Can you work these out from the model? Positions are in its coordinate system, mm. Face numbers are marked on the shaded views. Round coordinates to 2 decimals unless told otherwise and drop trailing zeros. Order: outer loops, then holes, each group sorted by start corner. A loop starts at its lowest first (then second) coordinate and runs counter-clockwise, first axis right, second up. Notation, with made-up numbers: (54.5, -10) -> (106.5, -10) arc R8 ccw to (106.5, -2) -> close; hole circle Ø9 at (52, -8.5). An arc over 180 degrees is marked (long way). Use a Markdown table: item, result. Add a question column.
Q1. I'm going to push flat-ended pins straight in: pin 1 Ø2 at (x, y) = (25.575, -43.247) entering from +Z (1 decimal); pin 2 Ø10 at (x, y) = (13, -30) entering from +Z; pin 3 Ø2 at (x, z) = (15, 4.5) entering from +Y. Where does each tip first touch, or does it pass through?
Q2. I need wall thicknesses on line 1 along X through (y, z) = (34.5, 5.5) (3 decimals); line 2 along X through (y, z) = (56.5, 3.25) (3 decimals); line 3 along X through (y, z) = (22.5, 3.5) (3 decimals). Which ranges of each line are inside material? Lowest first, please. Write a range as [from, to].
Q3. If we section it at D-D on z = 2: Give the number of separate pieces and of enclosed holes in the cut face, plus the area to 3 significant figures.
Q4. If we section it at C-C on x = -13: List the corners of the cut face in (y, z) for me.
Q5. If we section it at A-A on x = -3: List the corners of the cut face in (y, z) for me, plus the area to 3 significant figures.
Q6. We'd pull the mould along X, two halves only. Please class the marked faces 1 and 2: +X half, -X half, draft (parallel to the pull), parting line (faces both ways), or undercut.
Q7. If we section it at B-B on y = -59: List the corners of the cut face in (x, z) for me (3 decimals).
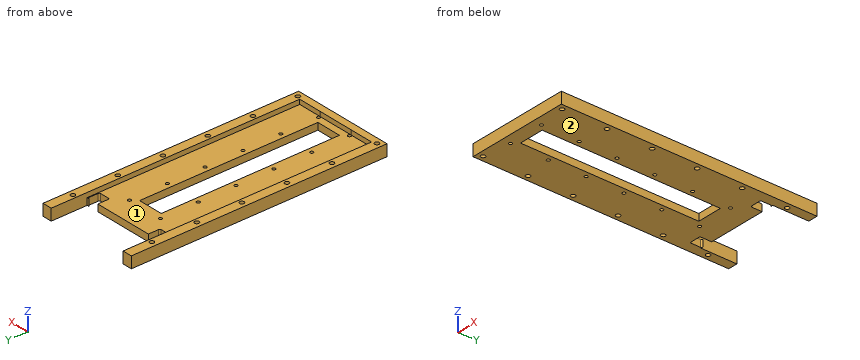
```python
from build123d import *

# Parameters (mm, degrees)
SKETCH1_W                 = 57.15
SKETCH1_H                 = 142.494
BOSS_EXTRUDE1_DEPTH       = 6.35
SKETCH2_W                 = 14
SKETCH2_H                 = 99
CUT_EXTRUDE1_DEPTH        = 78.025892621
SKETCH3_R                 = 1.2192
CUT_EXTRUDE2_DEPTH        = 78.025892621
LPATTERN1_COUNT           = 6
LPATTERN1_PITCH           = 25
LPATTERN1_COPY_1_SKETCH_R = 1.2192
LPATTERN1_COPY_1_DEPTH    = 78.025892621
LPATTERN1_COPY_2_SKETCH_R = 1.2192
LPATTERN1_COPY_2_DEPTH    = 78.025892621
LPATTERN1_COPY_3_SKETCH_R = 1.2192
LPATTERN1_COPY_3_DEPTH    = 78.025892621
LPATTERN1_COPY_4_SKETCH_R = 1.2192
LPATTERN1_COPY_4_DEPTH    = 78.025892621
LPATTERN1_COPY_5_SKETCH_R = 1.2192
LPATTERN1_COPY_5_DEPTH    = 78.025892621
SKETCH4_R                 = 0.889
CUT_EXTRUDE3_DEPTH        = 78.025892621
LPATTERN2_COUNT           = 6
LPATTERN2_PITCH           = 21
LPATTERN2_COPY_1_SKETCH_R = 0.889
LPATTERN2_COPY_1_DEPTH    = 78.025892621
LPATTERN2_COPY_2_SKETCH_R = 0.889
LPATTERN2_COPY_2_DEPTH    = 78.025892621
LPATTERN2_COPY_3_SKETCH_R = 0.889
LPATTERN2_COPY_3_DEPTH    = 78.025892621
LPATTERN2_COPY_4_SKETCH_R = 0.889
LPATTERN2_COPY_4_DEPTH    = 78.025892621
LPATTERN2_COPY_5_SKETCH_R = 0.889
LPATTERN2_COPY_5_DEPTH    = 78.025892621
SKETCH6_W                 = 41.91
SKETCH6_H                 = 10.16
CUT_EXTRUDE4_DEPTH        = 78.025892621
SKETCH8_W                 = 46.5
SKETCH8_H                 = 152.4
CUT_EXTRUDE6_DEPTH        = 2.54
SKETCH9_W                 = 57.15
SKETCH9_H                 = 6.35
CUT_EXTRUDE7_DEPTH        = 0.5
SKETCH11_W                = 6.5
SKETCH11_H                = 6.5
CUT_EXTRUDE8_DEPTH        = 78.025892621
FILLET1_R                 = 0.75
FILLET1_OF_MIRROR4_R      = 0.75
SKETCH12_W                = 41.91
SKETCH12_H                = 9.793222615
CUT_EXTRUDE9_DEPTH        = 77.858192368
SKETCH13_W                = 46.5
SKETCH13_H                = 19.953222615
CUT_EXTRUDE10_DEPTH       = 77.858192368


with BuildPart() as part:
    # Sketch1 → Boss-Extrude1 (new body)
    with BuildSketch(Plane.XY):
        Rectangle(SKETCH1_W, SKETCH1_H)
    extrude(amount=BOSS_EXTRUDE1_DEPTH)

    # Sketch2 → Cut-Extrude1 (cut, through all)
    with BuildSketch(Plane.XY.offset(6.35)):
        with Locations((0, -13.879757445)):
            Rectangle(SKETCH2_W, SKETCH2_H)
    extrude(amount=-CUT_EXTRUDE1_DEPTH, mode=Mode.SUBTRACT)

    # Sketch3 → Cut-Extrude2 (cut, through all)
    with BuildSketch(Plane.XY.offset(6.35)):
        with Locations((-25.575, -68.247)):
            Circle(SKETCH3_R)
    cut_extrude2 = extrude(amount=-CUT_EXTRUDE2_DEPTH, mode=Mode.SUBTRACT)

    # Mirror1: Cut-Extrude2 across plane
    add(cut_extrude2.mirror(Plane(origin=(0, 0, 0), x_dir=(0, 0, 1), z_dir=(1, 0, 0))), mode=Mode.SUBTRACT)

    # LPattern1: Cut-Extrude2 ×6
    with Locations(*[(0, i * LPATTERN1_PITCH, 0) for i in range(1, LPATTERN1_COUNT)]):
        add(cut_extrude2, mode=Mode.SUBTRACT)

    # LPattern1 copy 1 sketch → LPattern1 copy 1 (cut, through all)
    with BuildSketch(Plane(origin=(0, 25, 6.35), x_dir=(-1, 0, 0), z_dir=(0, 0, 1))):
        with Locations((-25.575, 68.247)):
            Circle(LPATTERN1_COPY_1_SKETCH_R)
    extrude(amount=-LPATTERN1_COPY_1_DEPTH, mode=Mode.SUBTRACT)

    # LPattern1 copy 2 sketch → LPattern1 copy 2 (cut, through all)
    with BuildSketch(Plane(origin=(0, 50, 6.35), x_dir=(-1, 0, 0), z_dir=(0, 0, 1))):
        with Locations((-25.575, 68.247)):
            Circle(LPATTERN1_COPY_2_SKETCH_R)
    extrude(amount=-LPATTERN1_COPY_2_DEPTH, mode=Mode.SUBTRACT)

    # LPattern1 copy 3 sketch → LPattern1 copy 3 (cut, through all)
    with BuildSketch(Plane(origin=(0, 75, 6.35), x_dir=(-1, 0, 0), z_dir=(0, 0, 1))):
        with Locations((-25.575, 68.247)):
            Circle(LPATTERN1_COPY_3_SKETCH_R)
    extrude(amount=-LPATTERN1_COPY_3_DEPTH, mode=Mode.SUBTRACT)

    # LPattern1 copy 4 sketch → LPattern1 copy 4 (cut, through all)
    with BuildSketch(Plane(origin=(0, 100, 6.35), x_dir=(-1, 0, 0), z_dir=(0, 0, 1))):
        with Locations((-25.575, 68.247)):
            Circle(LPATTERN1_COPY_4_SKETCH_R)
    extrude(amount=-LPATTERN1_COPY_4_DEPTH, mode=Mode.SUBTRACT)

    # LPattern1 copy 5 sketch → LPattern1 copy 5 (cut, through all)
    with BuildSketch(Plane(origin=(0, 125, 6.35), x_dir=(-1, 0, 0), z_dir=(0, 0, 1))):
        with Locations((-25.575, 68.247)):
            Circle(LPATTERN1_COPY_5_SKETCH_R)
    extrude(amount=-LPATTERN1_COPY_5_DEPTH, mode=Mode.SUBTRACT)

    # Sketch4 → Cut-Extrude3 (cut, through all)
    with BuildSketch(Plane.XY.offset(6.35)):
        with Locations((-10, -66.379757445)):
            Circle(SKETCH4_R)
    cut_extrude3 = extrude(amount=-CUT_EXTRUDE3_DEPTH, mode=Mode.SUBTRACT)

    # Mirror2: Cut-Extrude3 across plane
    add(cut_extrude3.mirror(Plane(origin=(0, 0, 0), x_dir=(0, 0, 1), z_dir=(1, 0, 0))), mode=Mode.SUBTRACT)

    # LPattern2: Cut-Extrude3 ×6
    with Locations(*[(0, i * LPATTERN2_PITCH, 0) for i in range(1, LPATTERN2_COUNT)]):
        add(cut_extrude3, mode=Mode.SUBTRACT)

    # LPattern2 copy 1 sketch → LPattern2 copy 1 (cut, through all)
    with BuildSketch(Plane(origin=(0, 21, 6.35), x_dir=(-1, 0, 0), z_dir=(0, 0, 1))):
        with Locations((-10, 66.379757445)):
            Circle(LPATTERN2_COPY_1_SKETCH_R)
    extrude(amount=-LPATTERN2_COPY_1_DEPTH, mode=Mode.SUBTRACT)

    # LPattern2 copy 2 sketch → LPattern2 copy 2 (cut, through all)
    with BuildSketch(Plane(origin=(0, 42, 6.35), x_dir=(-1, 0, 0), z_dir=(0, 0, 1))):
        with Locations((-10, 66.379757445)):
            Circle(LPATTERN2_COPY_2_SKETCH_R)
    extrude(amount=-LPATTERN2_COPY_2_DEPTH, mode=Mode.SUBTRACT)

    # LPattern2 copy 3 sketch → LPattern2 copy 3 (cut, through all)
    with BuildSketch(Plane(origin=(0, 63, 6.35), x_dir=(-1, 0, 0), z_dir=(0, 0, 1))):
        with Locations((-10, 66.379757445)):
            Circle(LPATTERN2_COPY_3_SKETCH_R)
    extrude(amount=-LPATTERN2_COPY_3_DEPTH, mode=Mode.SUBTRACT)

    # LPattern2 copy 4 sketch → LPattern2 copy 4 (cut, through all)
    with BuildSketch(Plane(origin=(0, 84, 6.35), x_dir=(-1, 0, 0), z_dir=(0, 0, 1))):
        with Locations((-10, 66.379757445)):
            Circle(LPATTERN2_COPY_4_SKETCH_R)
    extrude(amount=-LPATTERN2_COPY_4_DEPTH, mode=Mode.SUBTRACT)

    # LPattern2 copy 5 sketch → LPattern2 copy 5 (cut, through all)
    with BuildSketch(Plane(origin=(0, 105, 6.35), x_dir=(-1, 0, 0), z_dir=(0, 0, 1))):
        with Locations((-10, 66.379757445)):
            Circle(LPATTERN2_COPY_5_SKETCH_R)
    extrude(amount=-LPATTERN2_COPY_5_DEPTH, mode=Mode.SUBTRACT)

    # Sketch6 → Cut-Extrude4 (cut, through all)
    with BuildSketch(Plane.XY.offset(6.35)):
        with Locations((0, 55.873777385)):
            Rectangle(SKETCH6_W, SKETCH6_H)
    extrude(amount=-CUT_EXTRUDE4_DEPTH, mode=Mode.SUBTRACT)

    # Sketch8 → Cut-Extrude6 (cut)
    with BuildSketch(Plane.XY.offset(6.35)):
        with Locations((0, 8.953)):
            Rectangle(SKETCH8_W, SKETCH8_H)
    extrude(amount=-CUT_EXTRUDE6_DEPTH, mode=Mode.SUBTRACT)

    # Sketch9 → Cut-Extrude7 (cut)
    with BuildSketch(Plane(origin=(0, 71.247, 0), x_dir=(1, 0, 0), z_dir=(0, 1, 0))):
        with Locations((0, -3.175)):
            Rectangle(SKETCH9_W, SKETCH9_H)
    extrude(amount=-CUT_EXTRUDE7_DEPTH, mode=Mode.SUBTRACT)

    # Sketch11 → Cut-Extrude8 (cut, through all)
    with BuildSketch(Plane(origin=(0, 0, 0), x_dir=(-1, 0, 0), z_dir=(0, 0, -1))):
        with Locations((-19.6, 47.543777385)):
            Rectangle(SKETCH11_W, SKETCH11_H)
    cut_extrude8 = extrude(amount=-CUT_EXTRUDE8_DEPTH, mode=Mode.SUBTRACT)

    # Fillet1
    fillet1_edges = [part.edges().sort_by_distance(p)[0] for p in [
        (16.35, 44.293777385, 1.905),
        (22.85, 44.293777385, 1.905),
        (22.85, 50.793777385, 1.905),
    ]]
    fillet(fillet1_edges, radius=FILLET1_R)

    # Mirror4: Cut-Extrude8 across plane
    add(cut_extrude8.mirror(Plane(origin=(0, 0, 0), x_dir=(0, 0, 1), z_dir=(1, 0, 0))), mode=Mode.SUBTRACT)

    # Fillet1 of Mirror4
    fillet1_of_mirror4_edges = [part.edges().sort_by_distance(p)[0] for p in [
        (-16.35, 44.293777385, 1.905),
        (-22.85, 44.293777385, 1.905),
        (-22.85, 50.793777385, 1.905),
    ]]
    fillet(fillet1_of_mirror4_edges, radius=FILLET1_OF_MIRROR4_R)

    # Sketch12 → Cut-Extrude9 (cut, through all)
    with BuildSketch(Plane.XY.offset(3.81)):
        with Locations((0, 65.850388693)):
            Rectangle(SKETCH12_W, SKETCH12_H)
    extrude(amount=-CUT_EXTRUDE9_DEPTH, mode=Mode.SUBTRACT)

    # Sketch13 → Cut-Extrude10 (cut, through all)
    with BuildSketch(Plane.XY.offset(3.81)):
        with Locations((0, 60.770388693)):
            Rectangle(SKETCH13_W, SKETCH13_H)
    extrude(amount=-CUT_EXTRUDE10_DEPTH, mode=Mode.SUBTRACT)


solid = part.part
```
Answer below:
| question | item | result |
|---|---|---|
| 1 | pin 1 | through |
| 1 | pin 2 | z = 3.81 |
| 1 | pin 3 | y = 50.79 |
| 2 | line 1 | [-28.575, -23.25], [23.25, 28.575] |
| 2 | line 2 | [-28.575, -26.768], [-24.382, -23.25], [23.25, 24.382], [26.768, 28.575] |
| 2 | line 3 | [-28.575, -7], [7, 28.575] |
| 3 | separate pieces | 1 |
| 3 | enclosed holes | 25 |
| 3 | area | 5,630 mm² |
| 4 | outline | (-71.25, 0) -> (50.79, 0) -> (50.79, 3.81) -> (-67.25, 3.81) -> (-67.25, 6.35) -> (-71.25, 6.35) -> close |
| 5 | outline | (-71.25, 0) -> (-63.38, 0) -> (-63.38, 3.81) -> (-67.25, 3.81) -> (-67.25, 6.35) -> (-71.25, 6.35) -> close; (35.62, 0) -> (50.79, 0) -> (50.79, 3.81) -> (35.62, 3.81) -> close |
| 5 | area | 97.9 mm² |
| 6 | face 1 | undercut |
| 6 | face 2 | draft |
| 7 | outline | (-28.575, 0) -> (-7, 0) -> (-7, 3.81) -> (-23.25, 3.81) -> (-23.25, 6.35) -> (-28.575, 6.35) -> close; (7, 0) -> (28.575, 0) -> (28.575, 6.35) -> (23.25, 6.35) -> (23.25, 3.81) -> (7, 3.81) -> close |
